from build123d import *

# Parameters (mm, degrees)
SKETCH_1_W          = 24
SKETCH_1_H          = 16
EXTRUDE_1_DEPTH     = 12
SKETCH_2_W          = 33
SKETCH_2_H          = 12
EXTRUDE_2_DEPTH     = 2
SKETCH_3_R          = 1
CUT_EXTRUDE_1_DEPTH = 2
SKETCH_4_W          = 23
SKETCH_4_H          = 12
EXTRUDE_3_DEPTH     = 2
EXTRUDE_4_DEPTH     = 3
SKETCH_7_R          = 1.3
EXTRUDE_5_DEPTH     = 4


with BuildPart() as part:
    # 草图1 → 凸台-拉伸1 (new body)
    with BuildSketch(Plane(origin=(0, 0, 0), x_dir=(1, 0, 0), z_dir=(0, 1, 0))):
        Rectangle(SKETCH_1_W, SKETCH_1_H)
    extrude(amount=EXTRUDE_1_DEPTH)

    # 草图2 → 凸台-拉伸2 (add)
    with BuildSketch(Plane.XY.offset(8)):
        with Locations((0, 6)):
            Rectangle(SKETCH_2_W, SKETCH_2_H)
    extrude(amount=EXTRUDE_2_DEPTH)

    # 草图3 → 切除-拉伸1 (cut)
    with BuildSketch(Plane(origin=(0, 0, 8), x_dir=(-1, 0, 0), z_dir=(0, 0, -1))):
        with Locations((14.25, 6)):
            Circle(SKETCH_3_R)
        with Locations((-14.25, 6)):
            Circle(SKETCH_3_R)
    extrude(amount=-CUT_EXTRUDE_1_DEPTH, mode=Mode.SUBTRACT)

    # 草图4 → 凸台-拉伸3 (add)
    with BuildSketch(Plane.XY.offset(10)):
        with Locations((0, 6)):
            Rectangle(SKETCH_4_W, SKETCH_4_H)
    extrude(amount=EXTRUDE_3_DEPTH)

    # 草图6 → 凸台-拉伸4 (add)
    with BuildSketch(Plane.XY.offset(12)):
        with BuildLine():
            ThreePointArc((3.605751042, 4.7816434), (7.191817621, 6), (3.605751042, 7.2183566))
            ThreePointArc((3.605751042, 7.2183566), (1.230761216, 6), (3.605751042, 4.7816434))
        make_face()
    extrude(amount=EXTRUDE_4_DEPTH)

    # 草图7 → 凸台-拉伸5 (add)
    with BuildSketch(Plane.XY.offset(15)):
        with Locations((5.191817621, 6)):
            Circle(SKETCH_7_R)
    extrude(amount=EXTRUDE_5_DEPTH)


solid = part.part
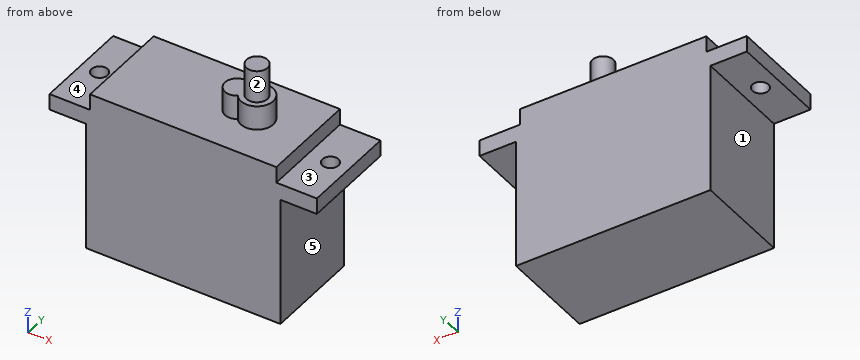
Work out the finished part from the listing and answer in its coordinate system (mm). Face numbers are marked on the shaded views. A direction names the side the tool comes from. Round coordinates to 2 decimals unless told otherwise and drop trailing zeros. Write each loop counter-clockwise with the first axis right and the second up, starting at its lowest first coordinate (ties: lowest second). Pieces come first, ordered by that corner, then holes. Notation, with made-up numbers: (86.25, 25) -> (106.25, 25) arc R22 cw to (106.25, 54) -> close; hole circle Ø2 at (31.5, -8.75). An arc over 180 degrees is marked (long way). Answer as CSV lines item,"result". Start each with the question number.
(1) A tool of negligible diameter and unlimited length cuts with its end or side. For the marked faces 1, 2, 3, 4 and 5, from which of +Z, -Z, +X, -X, +Y, -Y can it reach the whole face along a straight path? Write none if from no direction.
(2) Each of these flat-tipped pins is pushed along its axis until it touches: pin 1 (6 mm diameter, centred on x = 0, y = 5.5, fed in from +Z); pin 2 (5.5 mm diameter, centred on x = 15, y = 3.5, fed in from +Z); pin 3 (5 mm diameter, centred on x = 4.5, y = 4.5, fed in from +Z); pin 4 (6 mm diameter, centred on y = 8.5, z = 0, fed in from +X). Where does it stop, or does it pass through?
(3) Find the intervals of material crossed by probe 1 along Y at (x, z) = (14.25, 9.5); probe 2 along Z at (x, y) = (6.5, 6.5); probe 3 along Z at (x, y) = (-3.5, 10.25), in increasing order.
(4) The part is cut by section D-D, the plane z = -6. Give the vertices of the cut face in (x, y).
(5) The part is cut by section A-A, the plane x = -14.25. Give the vertices of the cut face in (y, z), then the cut area to 3 significant figures.
(6) The part is cut by section B-B, the plane y = 6. Give the vertices of the cut face in (x, z).
(7) The part is cut by section C-C, the plane x = 2.5. Give the vertices of the cut face in (y, z), then the cut area to 3 significant figures.
Output values:
1,face 1,"-Z, -X, +Y, -Y"
1,face 2,"+Z"
1,face 3,"+Z, +X, +Y, -Y"
1,face 4,"+Z, -X, +Y, -Y"
1,face 5,"-Z, +X, +Y, -Y"
2,pin 1,"stops at z = 15"
2,pin 2,"stops at z = 10"
2,pin 3,"stops at z = 19"
2,pin 4,"stops at x = 12"
3,probe 1,"y = 0 to 5, 7 to 12"
3,probe 2,"z = -8 to 15"
3,probe 3,"z = -8 to 12"
4,outline,"(-12, 0) -> (12, 0) -> (12, 12) -> (-12, 12) -> close"
5,outline,"(0, 8) -> (5, 8) -> (5, 10) -> (0, 10) -> close; (7, 8) -> (12, 8) -> (12, 10) -> (7, 10) -> close"
5,area,"20.0 mm²"
6,outline,"(-16.5, 8) -> (-15.25, 8) -> (-15.25, 10) -> (-16.5, 10) -> close; (-13.25, 8) -> (-12, 8) -> (-12, -8) -> (12, -8) -> (12, 8) -> (13.25, 8) -> (13.25, 10) -> (11.5, 10) -> (11.5, 12) -> (7.19, 12) -> (7.19, 15) -> (6.49, 15) -> (6.49, 19) -> (3.89, 19) -> (3.89, 15) -> (1.23, 15) -> (1.23, 12) -> (-11.5, 12) -> (-11.5, 10) -> (-13.25, 10) -> close; (15.25, 8) -> (16.5, 8) -> (16.5, 10) -> (15.25, 10) -> close"
7,outline,"(0, -8) -> (12, -8) -> (12, 12) -> (7.48, 12) -> (7.48, 15) -> (4.52, 15) -> (4.52, 12) -> (0, 12) -> close"
7,area,"249 mm²"
